CAD build for the part. Positions are in the model's coordinates, mm. Face numbers are marked on the shaded views. A direction names the side the tool comes from. Give positions to 0.01 mm unless a question says otherwise; leave off trailing zeros. Order: outer loops, then holes, each group sorted by start corner. A loop starts at its lowest first (then second) coordinate and runs counter-clockwise, first axis right, second up. Notation, with made-up numbers: (38.5, 51) -> (64.5, 51) arc R18 ccw to (64.5, 72) -> close; hole circle Ø5 at (40.5, 74.5). An arc over 180 degrees is marked (long way). Answer as CSV lines item,"result".
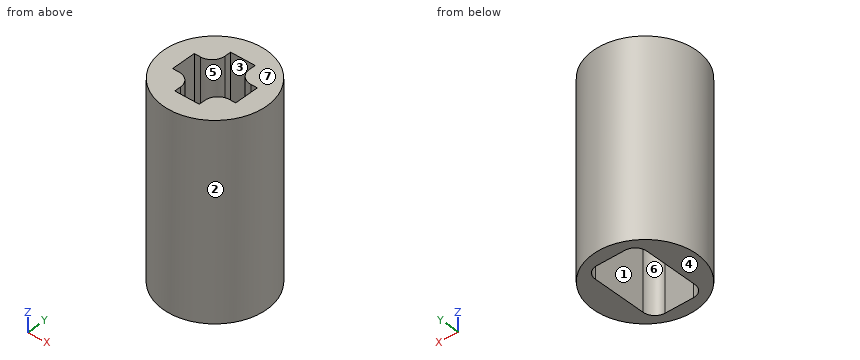
```python
from build123d import *

# Parameters (mm, degrees)
SKETCH1_R           = 4.5
BOSS_EXTRUDE1_DEPTH = 15
SKETCH2_W           = 4
SKETCH2_H           = 6
CUT_EXTRUDE1_DEPTH  = 7
CUT_EXTRUDE2_DEPTH  = 7
FILLET3_R           = 1
FILLET4_R           = 0.9
SKETCH4_R           = 4.5
SKETCH4_R_2         = 4
CUT_EXTRUDE3_DEPTH  = 15
SKETCH6_W           = 9.329019204
SKETCH6_H           = 8.683838676
SKETCH6_W_2         = 5
SKETCH6_H_2         = 7
CUT_EXTRUDE4_DEPTH  = 7
BOSS_EXTRUDE2_START = -15
SKETCH7_R           = 4
SKETCH7_R_2         = 3.5
BOSS_EXTRUDE2_DEPTH = 15
SKETCH8_W           = 7.8
SKETCH8_H           = 4.898979486
BOSS_EXTRUDE3_DEPTH = 1
SKETCH9_W           = 7.7
SKETCH9_H           = 5
BOSS_EXTRUDE4_DEPTH = 1
SKETCH10_R          = 4.498846738
SKETCH10_R_2        = 4
CUT_EXTRUDE7_DEPTH  = 21


with BuildPart() as part:
    # Sketch1 → Boss-Extrude1 (new body)
    with BuildSketch(Plane.XY):
        Circle(SKETCH1_R)
    extrude(amount=BOSS_EXTRUDE1_DEPTH)

    # Sketch2 → Cut-Extrude1 (cut)
    with BuildSketch(Plane(origin=(0, 0, 0), x_dir=(-1, 0, 0), z_dir=(0, 0, -1))):
        Rectangle(SKETCH2_W, SKETCH2_H)
    extrude(amount=-CUT_EXTRUDE1_DEPTH, mode=Mode.SUBTRACT)

    # Sketch3 → Cut-Extrude2 (cut)
    with BuildSketch(Plane.XY.offset(15)):
        Polygon((-0.95, -0.95), (-0.95, -2.45), (0.95, -2.45), (0.95, -0.95), (2.45, -0.95), (2.45, 0.95), (0.95, 0.95), (0.95, 2.45), (-0.95, 2.45), (-0.95, 0.95), (-2.45, 0.95), (-2.45, -0.95), align=None)
    extrude(amount=-CUT_EXTRUDE2_DEPTH, mode=Mode.SUBTRACT)

    # Fillet3
    fillet3_edges = [part.edges().sort_by_distance(p)[0] for p in [
        (0.95, -0.95, 11.5),
        (-0.95, -0.95, 11.5),
        (-0.95, 0.95, 11.5),
        (0.95, 0.95, 11.5),
    ]]
    fillet(fillet3_edges, radius=FILLET3_R)

    # Fillet4
    fillet4_edges = [part.edges().sort_by_distance(p)[0] for p in [
        (-2, 3, 3.5),
        (-2, -3, 3.5),
        (2, -3, 3.5),
        (2, 3, 3.5),
    ]]
    fillet(fillet4_edges, radius=FILLET4_R)

    # Sketch4 → Cut-Extrude3 (cut)
    with BuildSketch(Plane(origin=(0, 0, 0), x_dir=(-1, 0, 0), z_dir=(0, 0, -1))):
        Circle(SKETCH4_R)
        Circle(SKETCH4_R_2, mode=Mode.SUBTRACT)
    extrude(amount=-CUT_EXTRUDE3_DEPTH, mode=Mode.SUBTRACT)

    # Sketch6 → Cut-Extrude4 (cut)
    with BuildSketch(Plane(origin=(0, 0, 0), x_dir=(-1, 0, 0), z_dir=(0, 0, -1))):
        Rectangle(SKETCH6_W, SKETCH6_H)
        Rectangle(SKETCH6_W_2, SKETCH6_H_2, mode=Mode.SUBTRACT)
    extrude(amount=-CUT_EXTRUDE4_DEPTH, mode=Mode.SUBTRACT)

    # Sketch7 → Boss-Extrude2 (add)
    with BuildSketch(Plane.XY.offset(15).offset(BOSS_EXTRUDE2_START)):
        with Locations(Location((0, 0, 0), (0, 0, 180))):
            Circle(SKETCH7_R)
        Circle(SKETCH7_R_2, mode=Mode.SUBTRACT)
    extrude(amount=BOSS_EXTRUDE2_DEPTH)

    # Sketch8 → Boss-Extrude3 (add)
    with BuildSketch(Plane(origin=(2.5, 0, 0), x_dir=(0, 0, -1), z_dir=(1, 0, 0))):
        with Locations((-3.9, 0)):
            Rectangle(SKETCH8_W, SKETCH8_H)
    extrude(amount=BOSS_EXTRUDE3_DEPTH)

    # Sketch9 → Boss-Extrude4 (add)
    with BuildSketch(Plane.ZY.offset(2.5)):
        with Locations((3.85, -0.050510257)):
            Rectangle(SKETCH9_W, SKETCH9_H)
    extrude(amount=BOSS_EXTRUDE4_DEPTH)

    # Sketch10 → Cut-Extrude7 (cut)
    with BuildSketch(Plane(origin=(0, 0, 0), x_dir=(-1, 0, 0), z_dir=(0, 0, -1))):
        Circle(SKETCH10_R)
        Circle(SKETCH10_R_2, mode=Mode.SUBTRACT)
    extrude(amount=-CUT_EXTRUDE7_DEPTH, mode=Mode.SUBTRACT)


solid = part.part
```
1) Band-saw the part on D-D, the plane z = 10.25. Write the cut outline in (x, y), then the cut area to 3 significant figures.
Data:
outline,"circle Ø8 at (0, 0); hole (-2.45, -0.95) -> (-1.95, -0.95) arc R1 cw to (-0.95, -1.95) -> (-0.95, -2.45) -> (0.95, -2.45) -> (0.95, -1.95) arc R1 cw to (1.95, -0.95) -> (2.45, -0.95) -> (2.45, 0.95) -> (1.95, 0.95) arc R1 cw to (0.95, 1.95) -> (0.95, 2.45) -> (-0.95, 2.45) -> (-0.95, 1.95) arc R1 cw to (-1.95, 0.95) -> (-2.45, 0.95) -> close"
area,"34.4 mm2"
2) Pull direction X, two halves, no side cores. Call the marked faces 1, 2, 3 and 4: pulls with the +X half, pulls with the -X half, needs draft (parallel to the pull), parting line crosses it, or undercut.
Data:
face 1,"undercut"
face 2,"parting line crosses it"
face 3,"undercut"
face 4,"needs draft"
3) Pin check, flat tips, straight feed: P1, Ø1, axis at x = 3, z = 6, coming from the -Y side; P2, Ø1.5, axis at y = -1, z = 8.5, coming from the +X side; P3, Ø3, axis at x = -2, z = 2, coming from the -Y side. Stop position of each tip, or through.
Data:
P1,"stops at y = -3.12"
P2,"stops at x = 3.99"
P3,"stops at y = -3.97"
4) Band-saw the part on B-B, the plane x = 0. Write the cut outline in (y, z).
Data:
outline,"(-4, 0) -> (-3, 0) -> (-3, 7) -> (3, 7) -> (3, 0) -> (4, 0) -> (4, 15) -> (2.45, 15) -> (2.45, 8) -> (-2.45, 8) -> (-2.45, 15) -> (-4, 15) -> close"
5) Band-saw the part on C-C, the plane y = 0. Write the cut outline in (x, z), then the cut area to 3 significant figures.
Data:
outline,"(-4, 0) -> (-2, 0) -> (-2, 7) -> (2, 7) -> (2, 0) -> (4, 0) -> (4, 15) -> (2.45, 15) -> (2.45, 8) -> (-2.45, 8) -> (-2.45, 15) -> (-4, 15) -> close"
area,"57.7 mm2"
6) Which spindle directions (+Z, -Z, +X, -X, +Y, -Y) get a long thin tool onto all of the face, cutting with end or side? Do the marked faces 5, 6 and 7. Say none if no direction does.
Data:
face 5,"+Z"
face 6,"-Z"
face 7,"+Z, +X, -X, +Y, -Y"
7) Band-saw the part on A-A, the plane z = 5.5. Write the cut outline in (x, y), then the cut area to 3 significant figures.
Data:
outline,"circle Ø8 at (0, 0); hole (-2, -2.1) arc R0.9 ccw to (-1.1, -3) -> (1.1, -3) arc R0.9 ccw to (2, -2.1) -> (2, 2.1) arc R0.9 ccw to (1.1, 3) -> (-1.1, 3) arc R0.9 ccw to (-2, 2.1) -> close"
area,"27.0 mm2"
8) Wall check: line 1 along Y through (x, z) = (0, 10.5); line 2 along X through (y, z) = (-1.5, 2.5); line 3 along X through (y, z) = (-1.75, 3.5). Give the ranges that are in metal, low to high. Write a range as [from, to].
Data:
line 1,"y = [-4, -2.45], [2.45, 4]"
line 2,"x = [-3.71, -2], [2, 3.71]"
line 3,"x = [-3.6, -2], [2, 3.6]"
